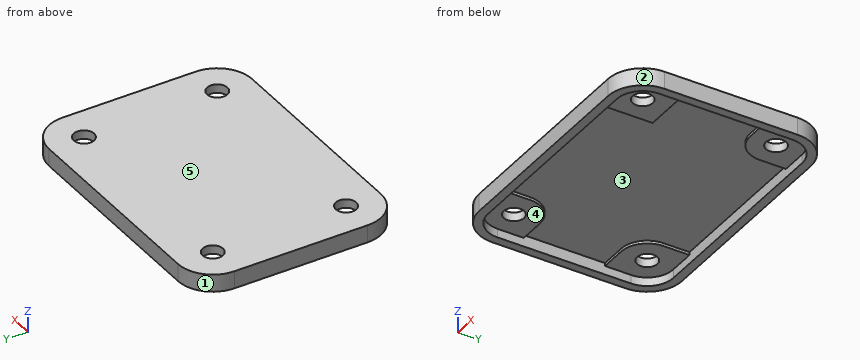
```python
from build123d import *

# Parameters (mm, degrees)
SKETCH1_R           = 1.75
BOSS_EXTRUDE1_DEPTH = 1.5
BOSS_EXTRUDE2_DEPTH = 1.5
SKETCH3_W           = 26.625
SKETCH3_H           = 13.95
CUT_EXTRUDE1_DEPTH  = 0.5


with BuildPart() as part:
    # Sketch1 → Boss-Extrude1 (new body)
    with BuildSketch(Plane.XY):
        with BuildLine():
            ThreePointArc((23.7625, 11.45), (22.012463018, 15.674963018), (17.7875, 17.425))
            Line((17.7875, 17.425), (-17.7875, 17.425))
            ThreePointArc((-17.7875, 17.425), (-22.012463018, 15.674963018), (-23.7625, 11.45))
            Line((-23.7625, 11.45), (-23.7625, -11.45))
            ThreePointArc((-23.7625, -11.45), (-22.012463018, -15.674963018), (-17.7875, -17.425))
            Line((-17.7875, -17.425), (17.7875, -17.425))
            ThreePointArc((17.7875, -17.425), (22.012463018, -15.674963018), (23.7625, -11.45))
            Line((23.7625, -11.45), (23.7625, 11.45))
        make_face()
        with Locations((-17.7875, -11.45)):
            Circle(SKETCH1_R, mode=Mode.SUBTRACT)
        with Locations((17.7875, -11.45)):
            Circle(SKETCH1_R, mode=Mode.SUBTRACT)
        with Locations((17.7875, 11.45)):
            Circle(SKETCH1_R, mode=Mode.SUBTRACT)
        with Locations((-17.7875, 11.45)):
            Circle(SKETCH1_R, mode=Mode.SUBTRACT)
    extrude(amount=BOSS_EXTRUDE1_DEPTH)

    # Sketch2 → Boss-Extrude2 (add)
    with BuildSketch(Plane(origin=(0, 0, 0), x_dir=(-1, 0, 0), z_dir=(0, 0, -1))):
        with BuildLine():
            Line((-17.7875, -17.425), (17.7875, -17.425))
            ThreePointArc((17.7875, -17.425), (22.012463018, -15.674963018), (23.7625, -11.45))
            Line((23.7625, -11.45), (23.7625, 11.45))
            ThreePointArc((23.7625, 11.45), (22.012463018, 15.674963018), (17.7875, 17.425))
            Line((17.7875, 17.425), (-17.7875, 17.425))
            ThreePointArc((-17.7875, 17.425), (-22.012463018, 15.674963018), (-23.7625, 11.45))
            Line((-23.7625, 11.45), (-23.7625, -11.45))
            ThreePointArc((-23.7625, -11.45), (-22.012463018, -15.674963018), (-17.7875, -17.425))
        make_face()
        with BuildLine():
            Line((17.7875, 15.925), (-17.7875, 15.925))
            ThreePointArc((-17.7875, 15.925), (-20.951802846, 14.614302846), (-22.2625, 11.45))
            Line((-22.2625, 11.45), (-22.2625, -11.45))
            ThreePointArc((-22.2625, -11.45), (-20.951802846, -14.614302846), (-17.7875, -15.925))
            Line((-17.7875, -15.925), (17.7875, -15.925))
            ThreePointArc((17.7875, -15.925), (20.951802846, -14.614302846), (22.2625, -11.45))
            Line((22.2625, -11.45), (22.2625, 11.45))
            ThreePointArc((22.2625, 11.45), (20.951802846, 14.614302846), (17.7875, 15.925))
        make_face(mode=Mode.SUBTRACT)
    extrude(amount=BOSS_EXTRUDE2_DEPTH)

    # Sketch3 → Cut-Extrude1 (cut)
    with BuildSketch(Plane(origin=(0, 0, 0), x_dir=(-1, 0, 0), z_dir=(0, 0, -1))):
        with BuildLine():
            Line((-17.7875, 6.975), (-13.3125, 6.975))
            Line((-13.3125, 6.975), (-13.3125, 11.45))
            ThreePointArc((-13.3125, 11.45), (-14.623197154, 8.285697154), (-17.7875, 6.975))
        make_face()
        Polygon((-17.787500036, -6.975), (-13.3125, -6.975), (-13.3125, 6.975), (-17.7875, 6.975), (-22.2625, 6.975), (-22.2625, -6.975), align=None)
        Polygon((-13.3125, 6.975), (13.3125, 6.975), (13.3125, 11.45), (13.3125, 15.925), (-13.3125, 15.925), (-13.3125, 11.45), align=None)
        with BuildLine():
            Line((13.3125, 6.975), (17.7875, 6.975))
            ThreePointArc((17.7875, 6.975), (14.623197154, 8.285697154), (13.3125, 11.45))
            Line((13.3125, 11.45), (13.3125, 6.975))
        make_face()
        Polygon((17.7875, -6.975), (22.2625, -6.975), (22.2625, 6.975), (17.7875, 6.975), (13.3125, 6.975), (13.3125, -6.975), align=None)
        with BuildLine():
            ThreePointArc((13.3125, -11.45), (14.623197154, -8.285697154), (17.7875, -6.975))
            Line((17.7875, -6.975), (13.3125, -6.975))
            Line((13.3125, -6.975), (13.3125, -11.45))
        make_face()
        Polygon((13.3125, -11.45), (13.3125, -6.975), (-13.3125, -6.975), (-13.3125, -11.45), (-13.3125, -15.925), (13.3125, -15.925), align=None)
        Rectangle(SKETCH3_W, SKETCH3_H)
    extrude(amount=-CUT_EXTRUDE1_DEPTH, mode=Mode.SUBTRACT)


solid = part.part
```
Geometry check sheet. Reference: the model listing, model coordinates, mm. Face numbers are marked on the shaded views. A direction names the side the tool comes from. Give positions to 0.01 mm unless a question says otherwise; leave off trailing zeros. Order: outer loops, then holes, each group sorted by start corner. A loop starts at its lowest first (then second) coordinate and runs counter-clockwise, first axis right, second up.
1. Section check C-C, the plane x = 11. Enter the section's corners in (y, z) (3 decimals).
2. Section check D-D, the plane x = 19. Enter the section's corners in (y, z) (3 decimals), and give its area (3 significant figures).
3. Access from +Z, -Z, +X, -X, +Y, -Y to the whole of each face (thin tool, end or side, straight path). Record for the marked faces 4 and 5.
4. Thickness scan on L1, parallel to Y at x = -4.5, z = -1 (3 decimals); L2, parallel to X at y = 2.5, z = 0.45; L3, parallel to X at y = 11, z = 1.05. Record the ranges inside material, lowest first.
5. Gauge pin test, flat ends, axial feed: pin 1 Ø8 at (x, y) = (18, -5) entering from -Z; pin 2 Ø0.6 at (y, z) = (-12, 0) entering from -X; pin 3 Ø6 at (x, y) = (4.5, 0) entering from -Z. Record the tip position at first contact, or that the pin passes through.
6. Release check for a two-part mould opening along Y. For the marked faces 1, 2 and 3 record: pulls with the +Y half, pulls with the -Y half, needs draft (parallel to the pull), parting line crosses it, or undercut.
7. Section check B-B, the plane y = -10.5. Enter the section's corners in (x, z).
Values follow:
1. outline: (-17.425, -1.5) - (-15.925, -1.5) - (-15.925, 0.5) - (15.925, 0.5) - (15.925, -1.5) - (17.425, -1.5) - (17.425, 1.5) - (-17.425, 1.5) - close
2. outline: (-17.301, -1.5) - (-15.758, -1.5) - (-15.758, 0) - (-12.712, 0) - (-12.712, 1.5) - (-17.301, 1.5) - close; (-10.188, 0) - (-6.975, 0) - (-6.975, 0.5) - (6.975, 0.5) - (6.975, 0) - (10.188, 0) - (10.188, 1.5) - (-10.188, 1.5) - close; (12.712, 0) - (15.758, 0) - (15.758, -1.5) - (17.301, -1.5) - (17.301, 1.5) - (12.712, 1.5) - close
2. area: 42.0 mm2
3. face 4: -Z
3. face 5: +Z, +X, -X, +Y, -Y
4. L1: y = -17.425 to -15.925, 15.925 to 17.425
4. L2: x = -23.76 to -22.26, 22.26 to 23.76
4. L3: x = -23.76 to -19.48, -16.1 to 16.1, 19.48 to 23.76
5. pin 1: stops at z = 0
5. pin 2: stops at x = -23.76
5. pin 3: stops at z = 0.5
6. face 1: pulls with the +Y half
6. face 2: pulls with the -Y half
6. face 3: undercut
7. outline: (-23.76, -1.5) - (-22.26, -1.5) - (-22.26, 0) - (-19.26, 0) - (-19.26, 1.5) - (-23.76, 1.5) - close; (-16.32, 0) - (-13.41, 0) - (-13.41, 0.5) - (13.31, 0.5) - (13.31, 0) - (16.32, 0) - (16.32, 1.5) - (-16.32, 1.5) - close; (19.26, 0) - (22.26, 0) - (22.26, -1.5) - (23.76, -1.5) - (23.76, 1.5) - (19.26, 1.5) - close
